Geometry check sheet. Reference: the model listing, model coordinates, mm. Face numbers are marked on the shaded views. A direction names the side the tool comes from. Give positions to 0.01 mm unless a question says otherwise; leave off trailing zeros. Order: outer loops, then holes, each group sorted by start corner. A loop starts at its lowest first (then second) coordinate and runs counter-clockwise, first axis right, second up. Notation, with made-up numbers: M 83.5,85.5 L 97.5,85.5 A12 ccw 97.5,93.5 Z; hole C -6.75,-6.5 d11. An arc over 180 degrees is marked long. Put each result on its own line as item: value. Start each with the question number.
Q1. Section check C-C on y = -30. Record the cut outline in (x, z).
Q2. Go/stop test with a flat-tipped pin: pin 1 (1 mm diameter, centred on x = 7.5, y = -27, fed in from +Z). Record where the tip stops, or that it passes through.
Q3. Section check B-B on x = -18. Record the cut outline in (y, z).
Q4. Section check D-D on x = -11. Record the cut outline in (y, z).
Q5. Section check A-A on z = -14. Record the cut outline in (x, y), then the cut area to 3 significant figures.
Q6. Material ranges on L1, parallel to Z at x = 23.5, y = -37; L2, parallel to X at y = -29.5, z = -17; L3, parallel to Z at x = 4.5, y = -35.5, recorded low to high.
Q7. Access from +Z, -Z, +X, -X, +Y, -Y to the whole of each face (thin tool, end or side, straight path). Record for the marked faces 1, 2 and 3.
Q8. Mould release check, pull along Y, two halves, no side actions. Record for the marked faces 4, 5, 6 and 7: +Y half, -Y half, draft (parallel to the pull), parting line (faces both ways), or undercut.
```python
from build123d import *

# Parameters (mm, degrees)
F0_W     = 50
F0_H     = 40
F1_DEPTH = 40
F3_DEPTH = 40.001
F5_DEPTH = 5
F6_DEPTH = 5
F7_DEPTH = 5


with BuildPart() as f1:
    # F0 (on Front) → F1 (new body)
    with BuildSketch(Plane.XZ):
        Rectangle(F0_W, F0_H)
    extrude(amount=F1_DEPTH)

    # F2 (on face) → F3 (cut, through all)
    with BuildSketch(Plane.XZ.offset(40)):
        Polygon((-20, -9.515879), (-8, -20), (8, -20), (20, -9.515879), (0, -9.515879), align=None)
    extrude(amount=-F3_DEPTH, mode=Mode.SUBTRACT)

    # F4 (on face) → F5 (join)
    with BuildSketch(Plane.XY.offset(20)):
        Polygon((-25, 0), (-25, -40), (-20, -40), (25, -5), (25, 0), align=None)
    extrude(amount=F5_DEPTH)

    # F4 (on face) → F6 (cut)
    with BuildSketch(Plane.XY.offset(20)):
        Polygon((25, -5), (-20, -40), (-11.85589, -40), (25, -11.334308), align=None)
    extrude(amount=-F6_DEPTH, mode=Mode.SUBTRACT)

    # F4 (on face) → F7 (cut)
    with BuildSketch(Plane.XY.offset(20)):
        Polygon((25, -19), (-1, -40), (25, -40), align=None)
    extrude(amount=-F7_DEPTH, mode=Mode.SUBTRACT)


solid = f1.part
```
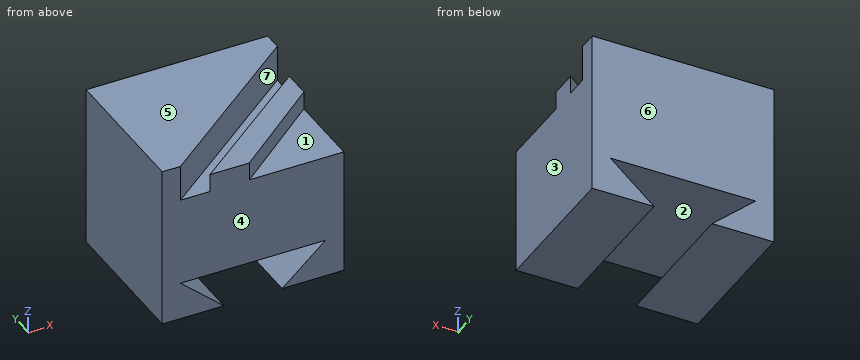
Results found:
1. outline: M -25,-20 L -8,-20 L -20,-9.52 L 20,-9.52 L 8,-20 L 25,-20 L 25,15 L 11.38,15 L 11.38,20 L 1,20 L 1,15 L -7.14,15 L -7.14,25 L -25,25 Z
2. pin 1: stops at z = 20
3. outline: M -40,-20 L 0,-20 L 0,-11.26 L -40,-11.26 Z; M -40,-9.52 L 0,-9.52 L 0,25 L -38.44,25 L -38.44,15 L -40,15 Z
4. outline: M -40,-20 L 0,-20 L 0,-17.38 L -40,-17.38 Z; M -40,-9.52 L 0,-9.52 L 0,25 L -33,25 L -33,15 L -39.33,15 L -39.33,20 L -40,20 Z
5. outline: M -25,-40 L -14.87,-40 L -14.87,0 L -25,0 Z; M 14.87,-40 L 25,-40 L 25,0 L 14.87,0 Z
5. area: 811 mm^2
6. L1: z = -20 to 15
6. L2: x = -25 to -11.43, 11.43 to 25
6. L3: z = -9.52 to 20
7. face 1: +Z, +X, -Y
7. face 2: +Y, -Y
7. face 3: +Z, -Z, +X, +Y, -Y
8. face 4: -Y half
8. face 5: draft
8. face 6: +Y half
8. face 7: undercut
